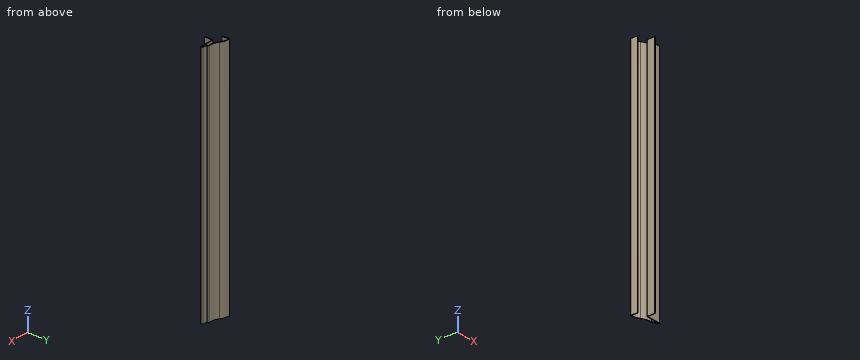
from build123d import *

# Parameters (mm, degrees)
EXTRUDE_THIN1_DEPTH = 333.375
FILLET1_R           = 1.016


with BuildPart() as part:
    # Sketch1 → Extrude-Thin1 (new body)
    with BuildSketch(Plane.XY):
        with BuildLine():
            Line((0, 0), (-0.396875, 9.921875))
            ThreePointArc((-0.396875, 9.921875), (6.266318546, 9.299504076), (12.303125, 6.411172093))
            ThreePointArc((12.303125, 6.411172093), (19.115525264, 3.32587731), (26.590625, 3.100654804))
            Line((26.590625, 3.100654804), (26.590625, 0.719404804))
            Line((26.590625, 0.719404804), (32.940625, -0.074345196))
            Line((32.940625, -0.074345196), (32.940625, -3.249345196))
            Line((32.940625, -3.249345196), (13.890625, -2.852470196))
            Line((13.890625, -2.852470196), (13.49375, -13.165191036))
            Line((13.49375, -13.165191036), (12.478501524, -13.126120189))
            Line((12.478501524, -13.126120189), (12.913764372, -1.815898471))
            Line((12.913764372, -1.815898471), (31.924625, -2.211958067))
            Line((31.924625, -2.211958067), (31.924625, -0.97125193))
            Line((31.924625, -0.97125193), (25.574625, -0.17750193))
            Line((25.574625, -0.17750193), (25.574625, 1.934694963))
            ThreePointArc((25.574625, 1.934694963), (18.305318895, 2.479849648), (11.710458333, 5.585943505))
            ThreePointArc((11.710458333, 5.585943505), (6.462301295, 8.184427992), (0.658241432, 8.964276082))
            Line((0.658241432, 8.964276082), (1.015188174, 0.040607527))
            Line((1.015188174, 0.040607527), (0, 0))
        make_face()
    extrude(amount=-EXTRUDE_THIN1_DEPTH)

    # Fillet1
    fillet1_edges = [part.edges().sort_by_distance(p)[0] for p in [
        (12.913764372, -1.815898471, -166.6875),
        (25.574625, -0.17750193, -166.6875),
        (-0.396875, 9.921875, -166.6875),
        (26.590625, 3.100654804, -166.6875),
        (32.940625, -0.074345196, -166.6875),
        (32.940625, -3.249345196, -166.6875),
    ]]
    fillet(fillet1_edges, radius=FILLET1_R)


solid = part.part
The listing builds one solid part. Answer for the finished solid, in the listing's coordinates (mm). Coordinates: 2 decimals unless noted, no trailing zeros. Write each loop counter-clockwise with the first axis right and the second up, starting at its lowest first coordinate (ties: lowest second). Pieces come first, ordered by that corner, then holes. Notation, with made-up numbers: M 34.25,70 L 65.25,70 A25 cw 65.25,96 Z; hole C 38,45 d1. An arc over 180 degrees is marked long. Use one line per item in the form item = value.
Item 1: Given P1, Ø1, axis at y = -1.5, z = -124, coming from the -X side; P2, Ø10, axis at y = -8, z = -182.5, coming from the -X side; P3, Ø1.5, axis at y = -9, z = -177, coming from the +X side, each flat-ended and moving along its own axis, determine where each tip first touches the part or whether it passes through.
Model answer:
P1 = 13.34
P2 = 12.48
P3 = 13.68
Item 2: Find section D-D, the plane x = 4. Give the vertices of the cut face in (y, z) (3 decimals).
Model answer:
outline = M 8.752,-333.375 L 9.78,-333.375 L 9.78,0 L 8.752,0 Z
Item 3: Find the intervals of material crossed by probe 1 along X at (y, z) = (1.5, -139); probe 2 along X at (y, z) = (-11.75, -257); probe 3 along X at (y, z) = (7.25, -215), in increasing order.
Model answer:
probe_1 = -0.06 to 0.96, 25.57 to 26.59
probe_2 = 12.53 to 13.55
probe_3 = -0.29 to 0.73, 8.88 to 11.03
Item 4: Find section C-C, the plane y = -8. Give the vertices of the cut face in (x, z) (3 decimals).
Model answer:
outline = M 12.676,-333.375 L 13.693,-333.375 L 13.693,0 L 12.676,0 Z
Item 5: Find section B-B, the plane z = -286. Give the vertices of the cut face in (x, y), plus the area to 3 significant figures.
Model answer:
outline = M -0.36,8.92 L 0,0 L 1.02,0.04 L 0.66,8.96 A18.03 cw 11.71,5.59 A20.07 ccw 25.57,1.93 L 25.57,0.72 A1.02 ccw 26.46,-0.29 L 31.92,-0.97 L 31.92,-2.21 L 13.91,-1.84 A1.02 ccw 12.88,-2.81 L 12.48,-13.13 L 13.49,-13.17 L 13.89,-2.85 L 31.9,-3.23 A1.02 ccw 32.94,-2.21 L 32.94,-0.97 A1.02 ccw 32.05,0.04 L 26.59,0.72 L 26.59,1.93 A1.02 ccw 25.47,2.94 A19.05 cw 12.3,6.41 A19.05 ccw 0.63,9.98 A1.02 ccw Z
area = 77.6 mm2
Item 6: Find section A-A, the plane x = 19.5. Give the vertices of the cut face in (y, z) (3 decimals).
Model answer:
outline = M -2.969,-333.375 L -1.953,-333.375 L -1.953,0 L -2.969,0 Z; M 2.204,-333.375 L 3.241,-333.375 L 3.241,0 L 2.204,0 Z
